The listing builds one solid part. Answer for the finished solid, in the listing's coordinates (mm). Face numbers are marked on the shaded views. A direction names the side the tool comes from. Coordinates: 2 decimals unless noted, no trailing zeros. Order: outer loops, then holes, each group sorted by start corner. A loop starts at its lowest first (then second) coordinate and runs counter-clockwise, first axis right, second up. Notation, with made-up numbers: (-16.5, 9.25) -> (21.5, 9.25) arc R17 cw to (21.5, 29.25) -> close; hole circle Ø10 at (23.5, -10.75). An arc over 180 degrees is marked (long way). Answer in a Markdown table with one row per item. Add a question column.
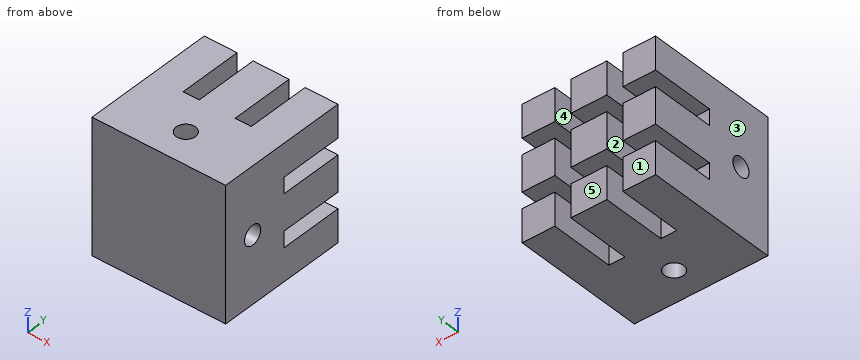
```python
from build123d import *

# Parameters (mm, degrees)
SKETCH2_W           = 26.416
SKETCH2_H           = 26.416
BOSS_EXTRUDE1_DEPTH = 26.416
SKETCH4_W           = 3.175
SKETCH4_H           = 26.416
SKETCH4_W_2         = 26.416
SKETCH4_H_2         = 3.175
CUT_EXTRUDE3_DEPTH  = 12.7
SKETCH7_R           = 1.905
CUT_EXTRUDE5_DEPTH  = 35.934004294
SKETCH8_R           = 1.905
CUT_EXTRUDE6_DEPTH  = 40.796215498


with BuildPart() as part:
    # Sketch2 → Boss-Extrude1 (new body)
    with BuildSketch(Plane.XY):
        with Locations((5.08, -0.508)):
            Rectangle(SKETCH2_W, SKETCH2_H)
    extrude(amount=-BOSS_EXTRUDE1_DEPTH)

    # Sketch4 → Cut-Extrude3 (cut)
    with BuildSketch(Plane(origin=(0, 12.7, 0), x_dir=(1, 0, 0), z_dir=(0, 1, 0))):
        with Locations((-0.0635, 13.208)):
            Rectangle(SKETCH4_W, SKETCH4_H)
        with Locations((10.2235, 13.208)):
            Rectangle(SKETCH4_W, SKETCH4_H)
        with Locations((5.08, 18.3515)):
            Rectangle(SKETCH4_W_2, SKETCH4_H_2)
        with Locations((5.08, 8.0645)):
            Rectangle(SKETCH4_W_2, SKETCH4_H_2)
    extrude(amount=-CUT_EXTRUDE3_DEPTH, mode=Mode.SUBTRACT)

    # Sketch7 → Cut-Extrude5 (cut, through all)
    with BuildSketch(Plane.XY):
        with Locations((5.08, -7.366)):
            Circle(SKETCH7_R)
    extrude(amount=-CUT_EXTRUDE5_DEPTH, mode=Mode.SUBTRACT)

    # Sketch8 → Cut-Extrude6 (cut, through all)
    with BuildSketch(Plane(origin=(18.288, 0, 0), x_dir=(0, 0, -1), z_dir=(1, 0, 0))):
        with Locations(Location((13.208, -7.366, 0), (0, 0, 90))):
            Circle(SKETCH8_R)
    extrude(amount=-CUT_EXTRUDE6_DEPTH, mode=Mode.SUBTRACT)


solid = part.part
```
Q1. A cutting plane is placed at B-B (y = 3.5). State how many separate pieces and enclosed holes the cut face has, then the cut area to 3 significant figures.
Q2. Straight lines are drawn through the part: line 1 (Z direction, x = 5.5, y = 1); line 2 (X direction, y = 5.5, z = -16.25); line 3 (Y direction, x = 5.08, z = -7.5). For each, find the intervals that lie inside material, in ascending order.
Q3. For the marked faces 4 and 5, determine the directions among +Z, -Z, +X, -X, +Y, -Y from which every point of the face is accessible in a straight line to the end or side of a thin tool.
Q4. Given pin 1 (3.5 mm diameter, centred on y = -7.366, z = -13.208, fed in from -X), flat-ended and moving along its own axis, determine where the tip first touches the part or whether it passes through.
Q5. Determine the mould class of the marked faces 1, 2 and 3 for opening direction X: +X half, -X half, draft (parallel to the pull), parting line (faces both ways), or undercut.
Q6. A cutting plane is placed at A-A (x = 0). Determine the outline of the cut face in (y, z) (3 decimals).
Q7. A cutting plane is placed at D-D (x = -5). Determine the outline of the cut face in (y, z) (3 decimals), then the cut area to 3 significant figures.
Q8. A cutting plane is placed at C-C (z = -2.5). Determine the outline of the cut face in (x, y) (3 decimals).
Returned:
| question | item | result |
|---|---|---|
| 1 | separate pieces | 9 |
| 1 | enclosed holes | 0 |
| 1 | area | 403 mm² |
| 2 | line 1 | z = -26.42 to -19.94, -16.76 to -9.65, -6.48 to 0 |
| 2 | line 2 | x = -8.13 to -1.65, 1.52 to 8.64, 11.81 to 18.29 |
| 2 | line 3 | y = -13.72 to -9.27, -5.46 to 0 |
| 3 | face 4 | +Z, -Z, +Y |
| 3 | face 5 | +Z, -Z, +X, -X, +Y |
| 4 | pin 1 | passes through |
| 5 | face 1 | draft |
| 5 | face 2 | undercut |
| 5 | face 3 | -X half |
| 6 | outline | (-13.716, -26.416) -> (0, -26.416) -> (0, 0) -> (-13.716, 0) -> close; hole circle Ø3.81 at (-7.366, -13.208) |
| 7 | outline | (-13.716, -26.416) -> (12.7, -26.416) -> (12.7, -19.939) -> (0, -19.939) -> (0, -16.764) -> (12.7, -16.764) -> (12.7, -9.652) -> (0, -9.652) -> (0, -6.477) -> (12.7, -6.477) -> (12.7, 0) -> (-13.716, 0) -> close; hole circle Ø3.81 at (-7.366, -13.208) |
| 7 | area | 606 mm² |
| 8 | outline | (-8.128, -13.716) -> (18.288, -13.716) -> (18.288, 12.7) -> (11.811, 12.7) -> (11.811, 0) -> (8.636, 0) -> (8.636, 12.7) -> (1.524, 12.7) -> (1.524, 0) -> (-1.651, 0) -> (-1.651, 12.7) -> (-8.128, 12.7) -> close; hole circle Ø3.81 at (5.08, -7.366) |
